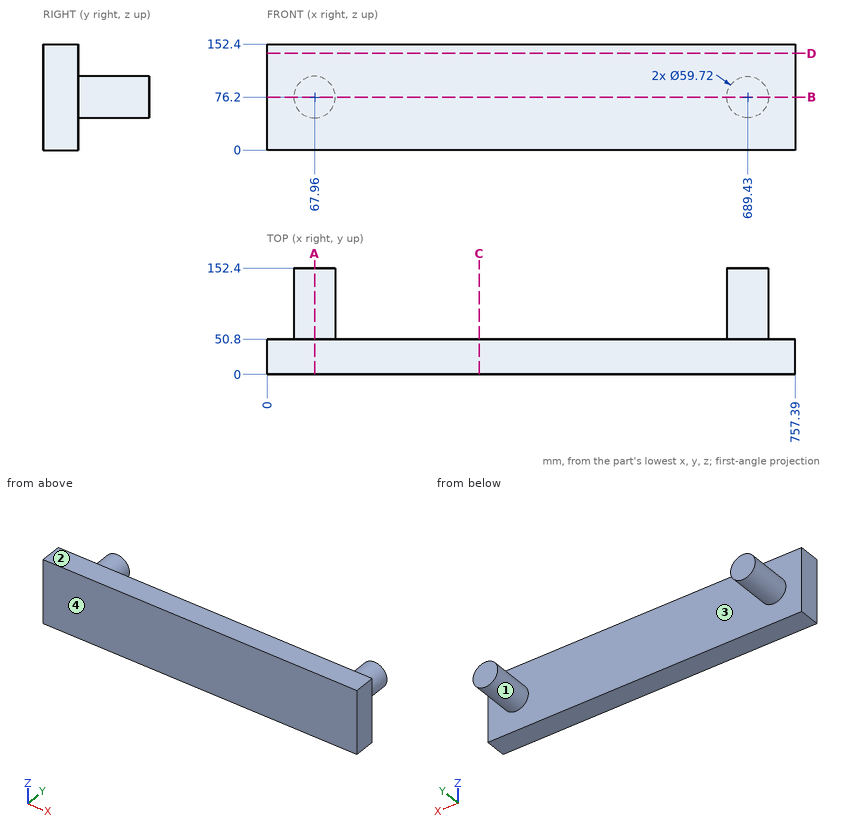
Part print with two shaded views. Sizes in mm from the minimum x, y, z corner. A direction names the side the tool comes from. Round coordinates to 2 decimals unless told otherwise and drop trailing zeros. Loops run counter-clockwise (first coordinate to the right, second up) from the corner with the lowest first, then second, coordinate; pieces in that order, holes last. Notation, with made-up numbers: M 79,70 L 95,70 A16 cw 95,75 Z; hole C 63.25,80.5 d1. An arc over 180 degrees is marked long. Put each result on its own line as item: value. Start each with the question number.
Item 1: Cut at B-B (z = 76.2). List the corners of the cut face in (x, y), then the cut area to 3 significant figures.
Item 2: Cut at D-D (z = 139). List the corners of the cut face in (x, y), then the cut area to 3 significant figures.
Item 3: Drill centre lines: line 1 along Y through (x, z) = (527.5, 94); line 2 along X through (y, z) = (70, 54.5); line 3 along X through (y, z) = (119.5, 92.5). Where is each one in solid material? Low to high.
Item 4: Mould opens along X. For the marked faces 3 and 4 say: released by +X, released by -X, zero draft, split by the parting line, or undercut.
Item 5: Drop flat-ended pins along their axis: P1, Ø1.5, axis at y = 65.5, z = 45, coming from the +X side; P2, Ø5, axis at y = 86.5, z = 68.5, coming from the +X side; P3, Ø4, axis at x = 98.5, z = 99.5, coming from the +Y side. Give the stop position or say it passes through.
Item 6: Cut at A-A (x = 67.96). List the corners of the cut face in (y, z), then the cut area to 3 significant figures.
Item 7: 3-axis set-ups, long thin cutter, end or side, ignore diameter. For the marked faces 1 and 2: which of +Z, -Z, +X, -X, +Y, -Y reach the whole face in a straight line?
Item 8: Cut at C-C (x = 304). List the corners of the cut face in (y, z), then the cut area to 3 significant figures.
Answer block:
1. outline: M 0,0 L 757.39,0 L 757.39,50.8 L 719.29,50.8 L 719.29,152.4 L 659.57,152.4 L 659.57,50.8 L 97.82,50.8 L 97.82,152.4 L 38.1,152.4 L 38.1,50.8 L 0,50.8 Z
1. area: 50,600 mm2
2. outline: M 0,0 L 757.39,0 L 757.39,50.8 L 0,50.8 Z
2. area: 38,500 mm2
3. line 1: 0 to 50.8
3. line 2: 47.45 to 88.47, 668.92 to 709.94
3. line 3: 42.94 to 92.98, 664.41 to 714.45
4. face 3: undercut
4. face 4: zero draft
5. P1: through
5. P2: x = 718.83
5. P3: y = 50.8
6. outline: M 0,0 L 50.8,0 L 50.8,46.34 L 152.4,46.34 L 152.4,106.06 L 50.8,106.06 L 50.8,152.4 L 0,152.4 Z
6. area: 13,800 mm2
7. face 1: +Y
7. face 2: +Z, +X, -X, +Y, -Y
8. outline: M 0,0 L 50.8,0 L 50.8,152.4 L 0,152.4 Z
8. area: 7,740 mm2
